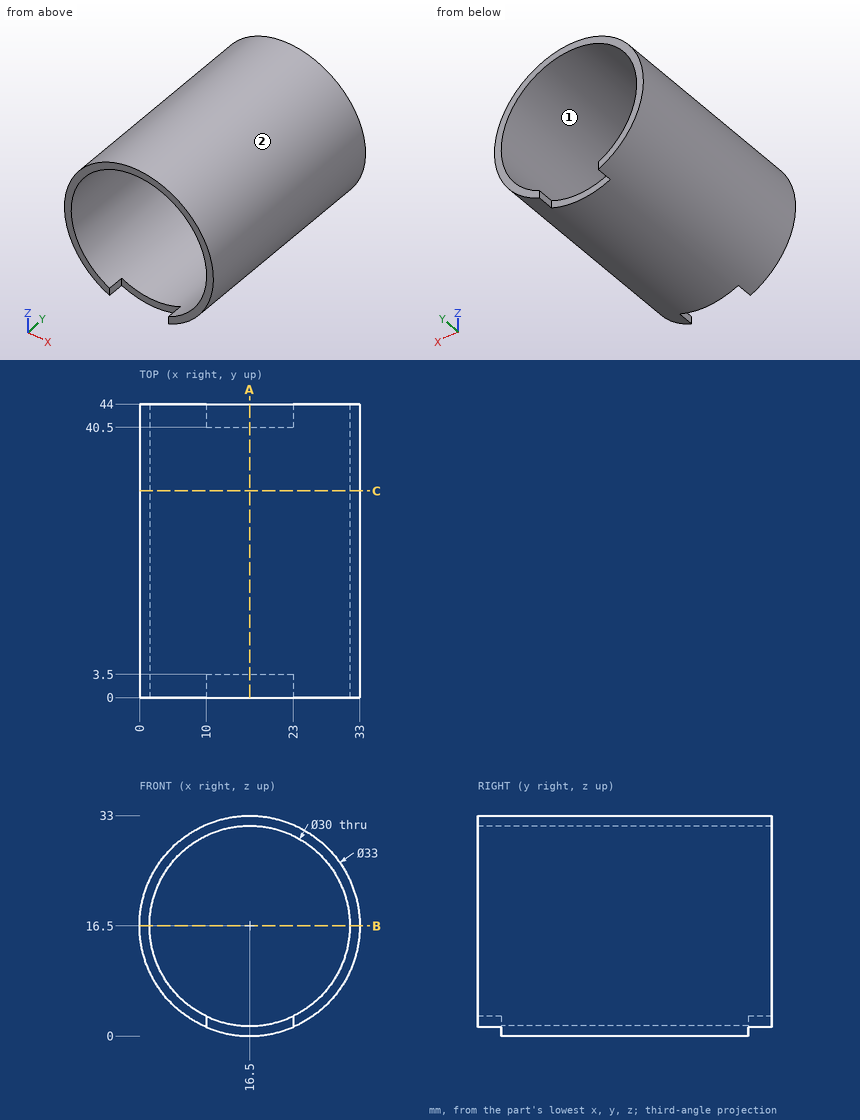
Geometry: see drawing. Coordinates: mm, zero at the bounding-box minimum. Coordinates: 2 decimals unless noted, no trailing zeros. Write each loop counter-clockwise with the first axis right and the second up, starting at its lowest first coordinate (ties: lowest second). Pieces come first, ordered by that corner, then holes. Notation, with made-up numbers: M 18.25,12.25 L 65.25,12.25 A15 ccw 65.25,20.25 Z; hole C 35,-5.75 d2. An arc over 180 degrees is marked long. Answer as a JSON object with one key per item and string values.
1. Cut plane C-C on y = 31. Output: boundary loops of the cut face in (x, z).
Evaluation:
{"outline": "C 16.5,16.5 d33; hole C 16.5,16.5 d30"}
2. Draft query along X for the marked faces 1 and 2. Return one class per face: released by +X, released by -X, zero draft, split by the parting line, or undercut.
Evaluation:
{"face 1": "undercut", "face 2": "split by the parting line"}
3. Cut plane B-B on z = 16.5. Output: boundary loops of the cut face in (x, y), plus the area to 3 significant figures.
Evaluation:
{"outline": "M 0,0 L 1.5,0 L 1.5,44 L 0,44 Z; M 31.5,0 L 33,0 L 33,44 L 31.5,44 Z", "area": "132 mm^2"}
4. Contact query for flat-ended pins moving along their axis: P1, Ø4, axis at y = 9.5, z = 3.5, coming from the -X side; P2, Ø0.8, axis at y = 2.5, z = 2, coming from the -X side; P3, Ø0.8, axis at y = 42.5, z = 2, coming from the +X side; P4, Ø18, axis at x = 16.5, z = 16.5, coming from the -Y side. Output: stop coordinate, or through.
Evaluation:
{"P1": "x = 4.2", "P2": "x = 7.93", "P3": "x = 25.07", "P4": "through"}
5. Cut plane A-A on x = 16.5. Output: boundary loops of the cut face in (y, z).
Evaluation:
{"outline": "M 0,31.5 L 44,31.5 L 44,33 L 0,33 Z; M 3.5,0 L 40.5,0 L 40.5,1.5 L 3.5,1.5 Z"}
6. Ray query, L1, parallel to X at y = 29, z = 16.5; L2, parallel to Z at x = 16, y = 31; L3, parallel to X at y = 39.5, z = 19. Return the intervals inside material, ascending.
Evaluation:
{"L1": "0 to 1.5, 31.5 to 33", "L2": "0.01 to 1.51, 31.49 to 32.99", "L3": "0.19 to 1.71, 31.29 to 32.81"}
